Part print with two shaded views. Sizes in mm from the minimum x, y, z corner. A direction names the side the tool comes from. Round coordinates to 2 decimals unless told otherwise and drop trailing zeros. Loops run counter-clockwise (first coordinate to the right, second up) from the corner with the lowest first, then second, coordinate; pieces in that order, holes last. Notation, with made-up numbers: (1.5, 78.5) -> (51.5, 78.5) arc R18 ccw to (51.5, 96.5) -> close; hole circle Ø8 at (89.5, 40.5). An arc over 180 degrees is marked (long way). Put each result on its own line as item: value. Start each with the question number.
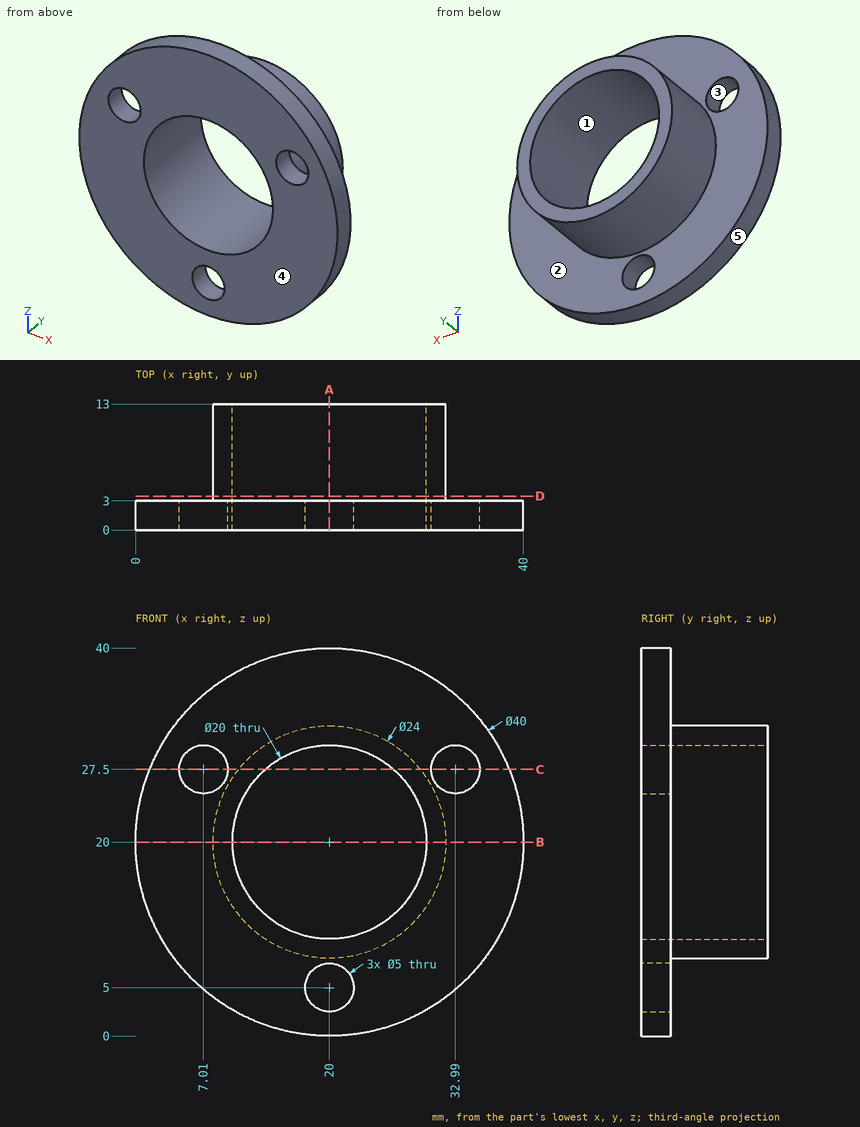
Item 1: Cut at C-C on z = 27.5. Write the cut outline in (x, y) (1 decimal).
Item 2: Cut at B-B on z = 20. Write the cut outline in (x, y).
Item 3: Wall check: line 1 (X direction, y = 2.05, z = 27.5) (1 decimal); line 2 (X direction, y = 6.5, z = 20); line 3 (Y direction, x = 15, z = 37.5). Give the ranges that are in metal, low to high. Write a range as from..to.
Item 4: Cut at D-D on y = 3.5. Write the cut outline in (x, z).
Item 5: 3-axis set-ups, long thin cutter, end or side, ignore diameter. For the marked faces 1 and 2: which of +Z, -Z, +X, -X, +Y, -Y reach the whole face in a straight line?
Item 6: Drop flat-ended pins along their axis: pin 1 (3 mm diameter, centred on y = 10, z = 21.5, fed in from -X); pin 2 (1.5 mm diameter, centred on x = 33.5, z = 36, fed in from -Y); pin 3 (2 mm diameter, centred on x = 17, z = 34, fed in from +Y); pin 4 (1 mm diameter, centred on y = 8.5, z = 13.5, fed in from -X). Give the stop position or say it passes through.
Item 7: Pull direction X, two halves, no side cores. Call the marked faces 3, 4 and 5: +X half, -X half, draft (parallel to the pull), parting line (faces both ways), or undercut.
Item 8: Cut at A-A on x = 20. Write the cut outline in (y, z).
Ans:
1. outline: (1.5, 0) -> (4.5, 0) -> (4.5, 3) -> (1.5, 3) -> close; (9.5, 0) -> (13.4, 0) -> (13.4, 13) -> (10.6, 13) -> (10.6, 3) -> (9.5, 3) -> close; (26.6, 0) -> (30.5, 0) -> (30.5, 3) -> (29.4, 3) -> (29.4, 13) -> (26.6, 13) -> close; (35.5, 0) -> (38.5, 0) -> (38.5, 3) -> (35.5, 3) -> close
2. outline: (0, 0) -> (10, 0) -> (10, 13) -> (8, 13) -> (8, 3) -> (0, 3) -> close; (30, 0) -> (40, 0) -> (40, 3) -> (32, 3) -> (32, 13) -> (30, 13) -> close
3. line 1: x = 1.5..4.5, 9.5..13.4, 26.6..30.5, 35.5..38.5
3. line 2: x = 8..10, 30..32
3. line 3: y = 0..3
4. outline: circle Ø24 at (20, 20); hole circle Ø20 at (20, 20)
5. face 1: +Y, -Y
5. face 2: +Y
6. pin 1: stops at x = 8
6. pin 2: passes through
6. pin 3: stops at y = 3
6. pin 4: stops at x = 9.61
7. face 3: undercut
7. face 4: draft
7. face 5: parting line
8. outline: (0, 0) -> (3, 0) -> (3, 2.5) -> (0, 2.5) -> close; (0, 7.5) -> (3, 7.5) -> (3, 8) -> (13, 8) -> (13, 10) -> (0, 10) -> close; (0, 30) -> (13, 30) -> (13, 32) -> (3, 32) -> (3, 40) -> (0, 40) -> close
